Check sheet for the modelled part. Datum: model origin and axes. Units: mm. A direction names the side the tool comes from. Coordinates: 2 decimals unless noted, no trailing zeros. One line per item, written item: value. Start each with the question number.
1) Draft check along Y on faces 1 (the flat face through (-37, 86, 2)), 2 (the flat face through (0, 100, 2)), 3 (the flat face through (-35, 42, 2)), 4 (the flat face through (-25, 62, 2)). Enter one of: +Y half, -Y half, draft (parallel to the pull), parting line (faces both ways), or undercut.
2) Sectioned sample at A-A on z = 2.4. Give the number of separate pieces and of enclosed holes in the cut face, plus the area to 3 significant figures.
3) Gauge pin test, flat ends, axial feed: P1, Ø5, axis at x = 40, y = 2, coming from the -Z side; P2, Ø1.8, axis at y = -65, z = 1.5, coming from the +X side. Record the tip position at first contact, or that the pin passes through.
4) Set-up check for faces 5 (the cylindrical face through (44.63, 31.82, 1.77)), 6 (the cylindrical face through (-25.513, 71.707, 1.774)), 7 (the flat face through (1, 0, 2)): record each of +Z, -Z, +X, -X, +Y, -Y from which the full face is reachable in a straight line by a thin tool's end or side.
5) Scan lines: line 1 along Y through (x, z) = (-40, 1.55); line 2 along Y through (x, z) = (18, 1.85); line 3 along Y through (x, z) = (8, 1.05). Record each from-to range of solid material in increasing order. Write a range as [from, to].
```python
from build123d import *

# Parameters (mm, degrees)
F0_R     = 1.5
F0_W     = 2.5
F0_H     = 22
F0_R_2   = 1.375
F1_DEPTH = 3.5
F2_R     = 5


# Not quite as in the source:
# - a feature names something its author has since deleted; it is built from what else it names


with BuildPart() as f1:
    # F0 (on Top) → F1 (new body)
    with BuildSketch(Plane.XY):
        with BuildLine():
            Line((-25, 52), (-45, 32))
            Line((-45, 32), (-45, -28))
            Line((-45, -28), (-25, -48))
            Line((-25, -48), (-25, -88))
            ThreePointArc((-25, -88), (-23.5355339059, -91.5355339059), (-20, -93))
            Line((-20, -93), (20, -93))
            ThreePointArc((20, -93), (23.5355339059, -91.5355339059), (25, -88))
            Line((25, -88), (25, -48))
            Line((25, -48), (45, -28))
            Line((45, -28), (45, 32))
            Line((45, 32), (25, 52))
            Line((25, 52), (25, 72))
            Line((25, 72), (37, 81))
            Line((37, 81), (37, 91))
            Line((37, 91), (25, 100))
            Line((25, 100), (-25, 100))
            Line((-25, 100), (-37, 91))
            Line((-37, 91), (-37, 81))
            Line((-37, 81), (-25, 72))
            Line((-25, 72), (-25, 52))
        make_face()
        with Locations((-20, -88)):
            Circle(F0_R, mode=Mode.SUBTRACT)
        with Locations((-8.5, -73.5)):
            Circle(F0_R, mode=Mode.SUBTRACT)
        with Locations((-40, -18)):
            Circle(F0_R, mode=Mode.SUBTRACT)
        with Locations((-40, 2)):
            Circle(F0_R, mode=Mode.SUBTRACT)
        with Locations((-31.75, 0)):
            Rectangle(F0_W, F0_H, mode=Mode.SUBTRACT)
        with Locations((-8.5, -34.5)):
            Circle(F0_R, mode=Mode.SUBTRACT)
        with Locations((-15, -10)):
            Circle(F0_R_2, mode=Mode.SUBTRACT)
        with Locations((0, -88)):
            Circle(F0_R, mode=Mode.SUBTRACT)
        with Locations((8, -73.5)):
            Circle(F0_R, mode=Mode.SUBTRACT)
        with Locations((20, -88)):
            Circle(F0_R, mode=Mode.SUBTRACT)
        with Locations((19, -34.5)):
            Circle(F0_R, mode=Mode.SUBTRACT)
        with Locations((18, -26.5)):
            Circle(F0_R, mode=Mode.SUBTRACT)
        with Locations((2.25, 0)):
            Rectangle(F0_W, F0_H, mode=Mode.SUBTRACT)
        with Locations((40, -18)):
            Circle(F0_R, mode=Mode.SUBTRACT)
        with Locations((40, 2)):
            Circle(F0_R, mode=Mode.SUBTRACT)
        with Locations((-40, 22)):
            Circle(F0_R, mode=Mode.SUBTRACT)
        with Locations((-15, 10)):
            Circle(F0_R_2, mode=Mode.SUBTRACT)
        with Locations((-21.5, 38)):
            Circle(F0_R, mode=Mode.SUBTRACT)
        with Locations((-32, 86)):
            Circle(F0_R_2, mode=Mode.SUBTRACT)
        with Locations((-20, 95)):
            Circle(F0_R, mode=Mode.SUBTRACT)
        with Locations((18, 16.5)):
            Circle(F0_R, mode=Mode.SUBTRACT)
        with Locations((21.5, 38)):
            Circle(F0_R, mode=Mode.SUBTRACT)
        with Locations((40, 22)):
            Circle(F0_R, mode=Mode.SUBTRACT)
        with Locations((0, 95)):
            Circle(F0_R, mode=Mode.SUBTRACT)
        with Locations((20, 95)):
            Circle(F0_R, mode=Mode.SUBTRACT)
        with Locations((32, 86)):
            Circle(F0_R_2, mode=Mode.SUBTRACT)
    extrude(amount=F1_DEPTH)

    # F2
    f2_edges = [f1.edges().sort_by_distance(p)[0] for p in [
        (-45, -28, 1.75),
        (-25, -48, 1.75),
        (25, -48, 1.75),
        (45, -28, 1.75),
        (45, 32, 1.75),
        (25, 52, 1.75),
        (25, 72, 1.75),
        (-25, 52, 1.75),
        (-45, 32, 1.75),
        (-25, 72, 1.75),
        (-37, 81, 1.75),
        (-37, 91, 1.75),
        (-25, 100, 1.75),
        (25, 100, 1.75),
        (37, 91, 1.75),
        (37, 81, 1.75),
    ]]
    fillet(f2_edges, radius=F2_R)


solid = f1.part
```
Answers:
1. face 1: draft
1. face 2: +Y half
1. face 3: undercut
1. face 4: undercut
2. separate pieces: 1
2. enclosed holes: 26
2. area: 13,000 mm2
3. P1: stops at z = 0
3. P2: stops at x = 25
4. face 5: +Z, -Z, +X, +Y
4. face 6: +Z, -Z, -X
4. face 7: +Z, -Z
5. line 1: y = [-33, -19.5], [-16.5, 0.5], [3.5, 20.5], [23.5, 37]
5. line 2: y = [-93, -35.62], [-33.38, -28], [-25, 15], [18, 100]
5. line 3: y = [-93, -75], [-72, 100]
